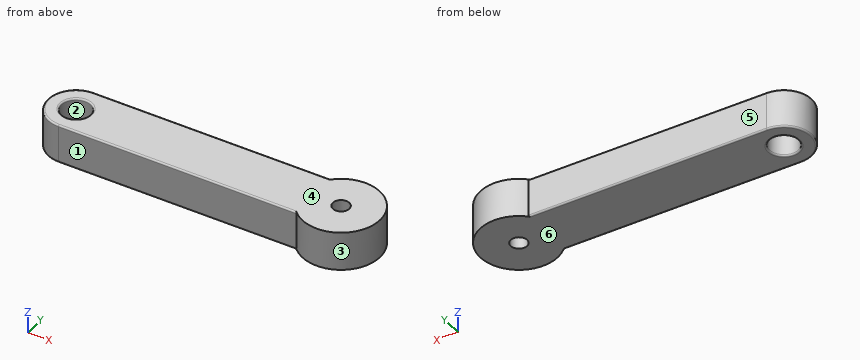
Autodesk Inventor part; units mm, degrees
ref_plane "YZ Plane" through (0, 0, 0) normal (1, 0, 0) x (0, 1, 0)
ref_plane "XZ Plane" through (0, 0, 0) normal (0, 1, 0) x (-1, 0, 0)
ref_plane "XY Plane" through (0, 0, 0) normal (0, 0, 1) x (1, 0, 0)
sketch "Sketch1" plane through (0, 0, 0) normal (0, 0, 1) x (1, 0, 0)
  circle A0 centre (0, 0) radius 4.7
  arc A1 (0, 9) -> (0, -9) centre (0, 0) ccw
  circle A2 centre (85, 0) radius 2.65
  arc A3 (76.3253, -9) -> (76.3253, 9) centre (85, 0) ccw
  line L0 (0, 9) -> (76.3253, 9)
  line L1 (0, -9) -> (76.3253, -9)
  dimension "d0" = 9.4
  dimension "d1" = 18
  dimension "d3" = 5.3
  dimension "d4" = 25
extrude "Extrusion1" add sketch "Sketch1" along normal blind 12.5
fillet "Fillet1" radius 0.5 8 edges at (-4.7, 0, 0) (-9, 0, 0) (38.1627, 9, 0) (38.1627, -9, 0) (-9, 0, 12.5) (38.1627, 9, 12.5) (38.1627, -9, 12.5) (-4.7, 0, 12.5)
properties part number "Arm Link Lower_3DPrint"
Can you work these out from the model? Positions are in its coordinate system, mm. Face numbers are marked on the shaded views. A direction names the side the tool comes from. Give positions to 0.01 mm unless a question says otherwise; leave off trailing zeros. Loops run counter-clockwise (first coordinate to the right, second up) from the corner with the lowest first, then second, coordinate; pieces in that order, holes last. Notation, with made-up numbers: M 72,87.5 L 115,87.5 A26 cw 115,106.5 Z; hole C -39,28 d2. An arc over 180 degrees is marked long. One line per item, written item: value.
1) Imagine slicing it at B-B on y = 0. Write out the boundary of the cut face in (x, z).
Geometry check:
outline: M -9,0.5 A0.5 ccw -8.5,0 L -5.2,0 A0.5 ccw -4.7,0.5 L -4.7,12 A0.5 ccw -5.2,12.5 L -8.5,12.5 A0.5 ccw -9,12 Z; M 4.7,0.5 A0.5 ccw 5.2,0 L 82.35,0 L 82.35,12.5 L 5.2,12.5 A0.5 ccw 4.7,12 Z; M 87.65,0 L 97.5,0 L 97.5,12.5 L 87.65,12.5 Z
2) Thinking about a two-plate mould opening in Y: for the marked faces 1, 2, 3 and 4, which applies, +Y half, -Y half, draft (parallel to the pull), parting line (faces both ways), or undercut?
Geometry check:
face 1: -Y half
face 2: undercut
face 3: parting line
face 4: draft
3) On a 3-axis mill with a long thin cutter (end or side, diameter ignored), from which of +Z, -Z, +X, -X, +Y, -Y can I reach the whole of each face in a straight line? I mean the marked faces 5 and 6. Say none if no direction works.
Geometry check:
face 5: +Z, -Z, -X, +Y
face 6: -Z, +X, -X, +Y, -Y
4) Imagine slicing it at A-A on x = 85. Write out the boundary of the cut face in (y, z).
Geometry check:
outline: M -12.5,0 L -2.65,0 L -2.65,12.5 L -12.5,12.5 Z; M 2.65,0 L 12.5,0 L 12.5,12.5 L 2.65,12.5 Z
5) Imagine slicing it at D-D on x = 61.5. Write out the boundary of the cut face in (y, z), and give its area (3 significant figures).
Geometry check:
outline: M -9,0.5 A0.5 ccw -8.5,0 L 8.5,0 A0.5 ccw 9,0.5 L 9,12 A0.5 ccw 8.5,12.5 L -8.5,12.5 A0.5 ccw -9,12 Z
area: 225 mm²
6) Imagine slicing it at C-C on z = 9.25. Write out the boundary of the cut face in (x, y).
Geometry check:
outline: M 0,-9 L 76.33,-9 A12.5 ccw long 76.33,9 L 0,9 A9 ccw Z; hole C 0,0 d9.4; hole C 85,0 d5.3
7) I'm going to push flat-ended pins straight in: pin 1 (3 mm diameter, centred on x = 14, z = 10, fed in from -Y); pin 2 (6 mm diameter, centred on x = 53.5, z = 8.5, fed in from +Y); pin 3 (1 mm diameter, centred on y = -6, z = 8, fed in from +X) (3 decimals). Where does each tip first touch, or does it pass through?
Geometry check:
pin 1: stops at y = -9
pin 2: stops at y = 9
pin 3: stops at x = 96.225
8) Please list where these lines run through material, in increasing order: line 1 (Y direction, x = 0, z = 8.75); line 2 (Y direction, x = 85, z = 5.75); line 3 (X direction, y = -1.5, z = 9.25).
Geometry check:
line 1: y = -9 to -4.7, 4.7 to 9
line 2: y = -12.5 to -2.65, 2.65 to 12.5
line 3: x = -8.87 to -4.45, 4.45 to 82.82, 87.18 to 97.41
